```python
from build123d import *

# Parameters (mm, degrees)
F0_W     = 55.88
F0_H     = 50.8
F1_DEPTH = 25.4
F2_R     = 13.97
F3_DEPTH = 127
F4_R     = 19.6578172959
F4_R_2   = 13.97
F5_DEPTH = 12.954


with BuildPart() as f1:
    # F0 (on Front) → F1 (new body, symmetric)
    with BuildSketch(Plane.XZ):
        Rectangle(F0_W, F0_H)
    extrude(amount=F1_DEPTH, both=True)

    # F2 (on face) → F3 (cut)
    with BuildSketch(Plane.XZ.offset(25.4)):
        Circle(F2_R)
    extrude(amount=-F3_DEPTH, mode=Mode.SUBTRACT)

    # F4 (on face) → F5 (join)
    with BuildSketch(Plane.XZ.offset(25.4)):
        Circle(F4_R)
        Circle(F4_R_2, mode=Mode.SUBTRACT)
    extrude(amount=F5_DEPTH)


solid = f1.part
```
Part model, mm, in its own coordinate system. A direction names the side the tool comes from. Round coordinates to 2 decimals unless told otherwise and drop trailing zeros. Loops run counter-clockwise (first coordinate to the right, second up) from the corner with the lowest first, then second, coordinate; pieces in that order, holes last.
1. Slice it at D-D (x = 21.5). Give the cut face in (y, z).
Solutions:
outline: (-25.4, -25.4) - (25.4, -25.4) - (25.4, 25.4) - (-25.4, 25.4) - close
2. Slice it at C-C (y = -20.5). Give the cut face in (x, z).
Solutions:
outline: (-27.94, -25.4) - (27.94, -25.4) - (27.94, 25.4) - (-27.94, 25.4) - close; hole circle Ø27.94 at (0, 0)
3. Flat gauge pins, fed straight in: pin 1 (1.5 mm diameter, centred on y = -30.5, z = 3.5, fed in from +X); pin 2 (1.5 mm diameter, centred on y = -31.5, z = 6, fed in from +X). Where does each tip first touch, or does it go through?
Solutions:
pin 1: stops at x = 19.46
pin 2: stops at x = 18.94
4. 3-axis set-ups, long thin cutter, end or side, ignore diameter. For faces 1 (the face through (-15.6, -31.79, -11.96)), 2 (the face through (0, 0, -25.4)): which of +Z, -Z, +X, -X, +Y, -Y reach the whole face in a straight line?
Solutions:
face 1: -Y
face 2: -Z, +X, -X, +Y, -Y
5. Slice it at A-A (z = 0). Give the cut face in (x, y).
Solutions:
outline: (-27.94, -25.4) - (-19.66, -25.4) - (-19.66, -38.35) - (-13.97, -38.35) - (-13.97, 25.4) - (-27.94, 25.4) - close; (13.97, -38.35) - (19.66, -38.35) - (19.66, -25.4) - (27.94, -25.4) - (27.94, 25.4) - (13.97, 25.4) - close
6. Drill centre lines: line 1 along Z through (x, y) = (0, 7.5); line 2 along Z through (x, y) = (0, -28); line 3 along Y through (x, z) = (-10, -19). Where is each one in solid material? Low to high.
Solutions:
line 1: z = -25.4 to -13.97, 13.97 to 25.4
line 2: z = -19.66 to -13.97, 13.97 to 19.66
line 3: y = -25.4 to 25.4
7. Slice it at B-B (x = -2). Give the cut face in (y, z), and give its area (3 significant figures).
Solutions:
outline: (-38.35, -19.56) - (-25.4, -19.56) - (-25.4, -25.4) - (25.4, -25.4) - (25.4, -13.83) - (-38.35, -13.83) - close; (-38.35, 13.83) - (25.4, 13.83) - (25.4, 25.4) - (-25.4, 25.4) - (-25.4, 19.56) - (-38.35, 19.56) - close
area: 1,320 mm2
